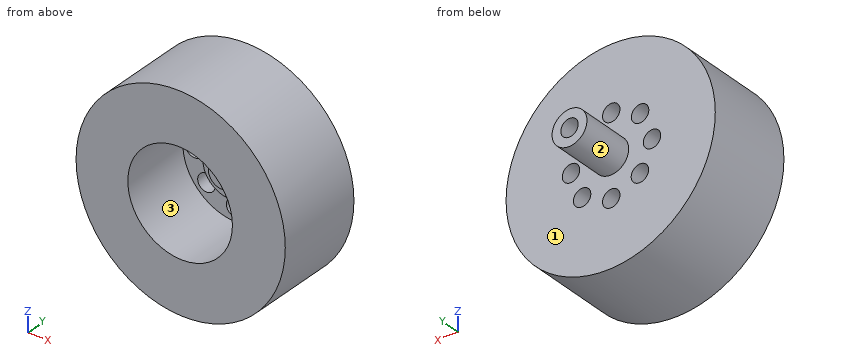
```python
from build123d import *

# Parameters (mm, degrees)
F0_R      = 19.05
F1_DEPTH  = 15.875
F2_R      = 9.525
F3_DEPTH  = 12.7
F4_R      = 1.5875
F5_DEPTH  = 25.4
F6_R      = 1.5875
F7_DEPTH  = 25.4
F8_R      = 1.5875
F9_DEPTH  = 25.4
F10_R     = 1.5875
F11_DEPTH = 25.4
F12_R     = 1.5875
F13_DEPTH = 25.4
F14_R     = 1.5875
F15_DEPTH = 25.4
F16_R     = 1.5875
F17_DEPTH = 25.4
F18_R     = 1.5875
F19_DEPTH = 25.4
F20_R     = 4.7625
F21_DEPTH = 1.5875
F22_R     = 2.38125
F23_DEPTH = 1.5875
F24_R     = 3.175
F25_DEPTH = 9.652
F26_R     = 1.5875
F27_DEPTH = 10.668


# Not quite as in the source:
# - a length typed as a fraction of an inch, garbled in the dataset ("3 / 203.2 mm" for 3/8 in), is restored


with BuildPart() as f1:
    # F0 (on Front) → F1 (new body)
    with BuildSketch(Plane.XZ):
        with Locations((0.1005562392, -0.0107518102)):
            Circle(F0_R)
    extrude(amount=F1_DEPTH)

    # F2 (on face) → F3 (cut)
    with BuildSketch(Plane.XZ.offset(15.875)):
        Circle(F2_R)
    extrude(amount=-F3_DEPTH, mode=Mode.SUBTRACT)

    # F4 (on face) → F5 (cut)
    with BuildSketch(Plane.XZ.offset(3.175)):
        with Locations((0, 7.3800315149)):
            Circle(F4_R)
    extrude(amount=-F5_DEPTH, mode=Mode.SUBTRACT)

    # F6 (on face) → F7 (cut)
    with BuildSketch(Plane.XZ.offset(3.175)):
        with Locations((0, -7.154897321)):
            Circle(F6_R)
    extrude(amount=-F7_DEPTH, mode=Mode.SUBTRACT)

    # F8 (on face) → F9 (cut)
    with BuildSketch(Plane.XZ.offset(3.175)):
        with Locations((7.3278159834, 0)):
            Circle(F8_R)
    extrude(amount=-F9_DEPTH, mode=Mode.SUBTRACT)

    # F10 (on face) → F11 (cut)
    with BuildSketch(Plane.XZ.offset(3.175)):
        with Locations((-7.4240518734, 0)):
            Circle(F10_R)
    extrude(amount=-F11_DEPTH, mode=Mode.SUBTRACT)

    # F12 (on face) → F13 (cut)
    with BuildSketch(Plane.XZ.offset(3.175)):
        with Locations((-5.2546598017, 5.1744827069)):
            Circle(F12_R)
    extrude(amount=-F13_DEPTH, mode=Mode.SUBTRACT)

    # F14 (on face) → F15 (cut)
    with BuildSketch(Plane.XZ.offset(3.175)):
        with Locations((5.3030503914, 4.8490739428)):
            Circle(F14_R)
    extrude(amount=-F15_DEPTH, mode=Mode.SUBTRACT)

    # F16 (on face) → F17 (cut)
    with BuildSketch(Plane.XZ.offset(3.175)):
        with Locations((-5.2185030654, -4.949348513)):
            Circle(F16_R)
    extrude(amount=-F17_DEPTH, mode=Mode.SUBTRACT)

    # F18 (on face) → F19 (cut)
    with BuildSketch(Plane.XZ.offset(3.175)):
        with Locations((5.3030503914, -4.9131917767)):
            Circle(F18_R)
    extrude(amount=-F19_DEPTH, mode=Mode.SUBTRACT)

    # F20 (on face) → F21 (join)
    with BuildSketch(Plane.XZ.offset(3.175)):
        with Locations((0.1396279233, 0.0120795696)):
            Circle(F20_R)
    extrude(amount=F21_DEPTH)

    # F22 (on face) → F23 (join)
    with BuildSketch(Plane.XZ.offset(4.7625)):
        Circle(F22_R)
    extrude(amount=F23_DEPTH)

    # F24 (on face) → F25 (join)
    with BuildSketch(Plane(origin=(0, 0, 0), x_dir=(-1, 0, 0), z_dir=(0, 1, 0))):
        Circle(F24_R)
    extrude(amount=F25_DEPTH)

    # F26 (on face) → F27 (cut)
    with BuildSketch(Plane(origin=(0, 9.652, 0), x_dir=(-1, 0, 0), z_dir=(0, 1, 0))):
        Circle(F26_R)
    extrude(amount=-F27_DEPTH, mode=Mode.SUBTRACT)


solid = f1.part
```
Geometry check sheet. Reference: the model listing, model coordinates, mm. Face numbers are marked on the shaded views. Coordinates: 2 decimals unless noted, no trailing zeros. Order: outer loops, then holes, each group sorted by start corner. A loop starts at its lowest first (then second) coordinate and runs counter-clockwise, first axis right, second up. Notation, with made-up numbers: (60.25, 86.25) - (78.25, 86.25) arc R30 ccw to (78.25, 110.25) - close; hole circle Ø11 at (79.25, 34.5). An arc over 180 degrees is marked (long way). Answer in a Markdown table with one row per item. Add a question column.
1. Material ranges on L1, parallel to Z at x = 0, y = -1.35; L2, parallel to X at y = -0.5, z = -4; L3, parallel to X at y = -0.25, z = -3.5, recorded low to high. Write a range as [from, to].
2. Section check D-D (z = -16.5). Enter the section's corners in (x, y) (3 decimals), plus the area to 3 significant figures.
3. Gauge pin test, flat ends, axial feed: pin 1 Ø3.5 at (x, z) = (7.33, 0) entering from +Y; pin 2 Ø1 at (y, z) = (-7, 3.5) entering from -X; pin 3 Ø10 at (y, z) = (-0.5, -13.5) entering from +X; pin 4 Ø3.5 at (x, z) = (-0.5, 0.5) entering from +Y. Record the tip position at first contact, or that the pin passes through.
4. Section check A-A (x = 1). Give the number of separate pieces and of enclosed holes in the cut face, plus the area to 3 significant figures.
5. Draft check along X on the marked faces 1, 2 and 3. Enter one of: +X half, -X half, draft (parallel to the pull), parting line (faces both ways), or undercut.
Data:
| question | item | result |
|---|---|---|
| 1 | L1 | z = [-19.06, -8.74], [-5.57, 5.79], [8.97, 19.04] |
| 1 | L2 | x = [-18.53, -6.49], [-3.95, 4], [6.6, 18.73] |
| 1 | L3 | x = [-18.63, -5.87], [-4.57, 4.58], [6.03, 18.83] |
| 2 | outline | (-9.439, -15.875) - (9.64, -15.875) - (9.64, 0) - (-9.439, 0) - close |
| 2 | area | 303 mm² |
| 3 | pin 1 | stops at y = 0 |
| 3 | pin 2 | stops at x = -18.71 |
| 3 | pin 3 | stops at x = 17.15 |
| 3 | pin 4 | stops at y = 9.65 |
| 4 | separate pieces | 3 |
| 4 | enclosed holes | 0 |
| 4 | area | 402 mm² |
| 5 | face 1 | draft |
| 5 | face 2 | parting line |
| 5 | face 3 | undercut |
